Autodesk Fusion 360 part; units mm, degrees
sketch "Skizze1" plane through (0, 0, 0) normal (0, 1, 0) x (1, 0, 0)
  line L0 (0.076, -28.1203) -> (3.2508, -24.9466)
  line L1 (3.2508, -24.9466) -> (39.9722, -24.9466)
  line L2 (39.9722, -24.9466) -> (39.9722, -3.2655)
  line L3 (39.9722, -3.2655) -> (43.147, -0.076)
  line L4 (43.147, -0.076) -> (61.7964, -0.076)
  line L5 (61.7964, -0.076) -> (65.6865, -4.3091)
  line L6 (65.6865, -4.3091) -> (65.6863, -51.4541)
  line L7 (65.6863, -51.4541) -> (62.5115, -54.6291)
  line L8 (62.5115, -54.6291) -> (3.2509, -54.6291)
  line L9 (3.2509, -54.6291) -> (0.0761, -51.4721)
  line L10 (0.0761, -51.4721) -> (0.076, -28.1203)
  circle A0 centre (6.1496, -29.6153) radius 2.4004
  circle A1 centre (20.857, -29.6153) radius 2.4004
  circle A2 centre (6.1496, -49.6141) radius 2.4004
  circle A3 centre (20.857, -49.6141) radius 2.4004
  circle A4 centre (55.5723, -32.7901) radius 2.4004
  circle A5 centre (56.1634, -9.2632) radius 2.4004
  circle A6 centre (6.1496, -29.6153) radius 1.5
  circle A7 centre (6.1496, -49.6141) radius 1.5
  circle A8 centre (20.857, -29.6153) radius 1.5
  circle A9 centre (20.857, -49.6141) radius 1.5
  circle A10 centre (56.1634, -9.2632) radius 1.5
  circle A11 centre (55.5723, -32.7901) radius 1.5
  point P0 (8.55, -29.6153)
  point P1 (23.2574, -29.6153)
  point P2 (8.55, -49.6141)
  point P3 (23.2574, -49.6141)
  point P4 (57.9727, -32.7901)
  point P5 (58.5638, -9.2632)
  dimension "d1" = 3
  dimension "d2" = 3
  dimension "d3" = 3
  dimension "d4" = 3
  dimension "d5" = 3
  dimension "d6" = 3
extrude "Extrusion1" add sketch "Skizze1" along normal blind 4 contours L0 L1 L2 L3 L4 L5 L6 L7 L8 L9 L10 | A0 | A1 | A2 | A3 | A4 | A5
sketch "Skizze2" plane through (0, 4, 0) normal (0, 1, 0) x (-1, 0, 0)
  circle A0 centre (-55.5723, 32.7901) radius 1.5
  circle A1 centre (-20.857, 49.6141) radius 1.5
  circle A2 centre (-20.857, 29.6153) radius 1.5
  circle A3 centre (-6.1496, 49.6141) radius 1.5
  circle A4 centre (-56.1634, 9.2632) radius 1.5
  circle A5 centre (-6.1496, 29.6153) radius 1.5
  line L0 (-0.0761, 51.4721) -> (-3.2509, 54.6291)
  line L1 (-3.2509, 54.6291) -> (-62.5115, 54.6291)
  line L2 (-62.5115, 54.6291) -> (-65.6863, 51.4541)
  line L3 (-65.6863, 51.4541) -> (-65.6865, 4.3091)
  line L4 (-65.6865, 4.3091) -> (-61.7964, 0.076)
  line L5 (-61.7964, 0.076) -> (-43.147, 0.076)
  line L6 (-43.147, 0.076) -> (-39.9722, 3.2655)
  line L7 (-39.9722, 3.2655) -> (-39.9722, 24.9466)
  line L8 (-39.9722, 24.9466) -> (-3.2508, 24.9466)
  line L9 (-3.2508, 24.9466) -> (-0.076, 28.1203)
  line L10 (-0.076, 28.1203) -> (-0.0761, 51.4721)
sketch "Skizze3" plane through (0, 4, 0) normal (0, 1, 0) x (-1, 0, 0)
Work out the finished part from the listing and answer in its coordinate system (mm). A direction names the side the tool comes from. Coordinates: 2 decimals unless noted, no trailing zeros. Loops run counter-clockwise (first coordinate to the right, second up) from the corner with the lowest first, then second, coordinate; pieces in that order, holes last. Notation, with made-up numbers: (42.25, -10) -> (50.25, -10) arc R13 ccw to (50.25, 5) -> close; hole circle Ø1 at (6.5, -26). An arc over 180 degrees is marked (long way). Write each question's results on one line, items separated by ' | '. Start each with the question number.
1) Find section B-B on z = 5. Determine the outline of the cut face in (x, y).
2) The mould has two halves that part along X. Classify faces 1 (the flat face through (64.12, 1.97, 53.02)), 2 (the cylindrical face through (5.82, 1.97, 48.15)), 3 (the flat face through (39.972, 2, 14)): pulls with the +X half, pulls with the -X half, needs draft (parallel to the pull), parting line crosses it, or undercut.
3) Consider line 1 along X through (y, z) = (2, 50); line 2 along Z through (x, y) = (13.5, 0.85); line 3 along X through (y, z) = (3.15, 10). Determine where each line is inside the solid, lowest interval first.
4) Flat-ended cylindrical pins translate along their axes: P1, Ø2, axis at y = 1.5, z = 11, coming from the -X side; P2, Ø1.2, axis at x = 20.5, y = 1.5, coming from the -Z side; P3, Ø3.5, axis at x = 55.57, z = 32.79, coming from the -Y side. Find the tip coordinate at first contact, or state that the pin passes through.
5) Find section A-A on y = 1.2. Determine the outline of the cut face in (x, z).
6) Find section C-C on x = 14. Determine the outline of the cut face in (y, z), then the cut area to 3 significant figures.
7) For faces 4 (the cylindrical face through (55.06, 1.97, 10.28)), 5 (the flat face through (21, 2, 24.947)), determine the directions among +Z, -Z, +X, -X, +Y, -Y from which every point of the face is accessible in a straight line to the end or side of a thin tool.
Response values:
1) outline: (39.97, 0) -> (65.69, 0) -> (65.69, 4) -> (39.97, 4) -> close
2) face 1: pulls with the +X half | face 2: undercut | face 3: pulls with the -X half
3) line 1: x = 0.08 to 4.7, 7.6 to 19.41, 22.31 to 65.69 | line 2: z = 24.95 to 54.63 | line 3: x = 39.97 to 54.86, 57.47 to 65.69
4) P1: stops at x = 39.97 | P2: stops at z = 24.95 | P3: stops at y = 0
5) outline: (0.08, 28.12) -> (3.25, 24.95) -> (39.97, 24.95) -> (39.97, 3.27) -> (43.15, 0.08) -> (61.8, 0.08) -> (65.69, 4.31) -> (65.69, 51.45) -> (62.51, 54.63) -> (3.25, 54.63) -> (0.08, 51.47) -> close; hole circle Ø3 at (6.15, 29.62); hole circle Ø3 at (6.15, 49.61); hole circle Ø3 at (20.86, 29.62); hole circle Ø3 at (20.86, 49.61); hole circle Ø3 at (55.57, 32.79); hole circle Ø3 at (56.16, 9.26)
6) outline: (0, 24.95) -> (4, 24.95) -> (4, 54.63) -> (0, 54.63) -> close | area: 119 mm^2
7) face 4: +Y, -Y | face 5: -Z, -X, +Y, -Y
